Input: dimensioned drawing with shaded views. Units: mm. Origin: part minimum x, y, z. Coordinates: 2 decimals unless noted, no trailing zeros. Order: outer loops, then holes, each group sorted by start corner. A loop starts at its lowest first (then second) coordinate and runs counter-clockwise, first axis right, second up. Notation, with made-up numbers: (18, 77.25) -> (65, 77.25) arc R26 ccw to (65, 91.25) -> close; hole circle Ø10 at (56, 71.5). An arc over 180 degrees is marked (long way). Answer in a Markdown table with one row per item. Add a question column.
1) Section query C-C on z = 39. Return the cut outline in (x, y), then the cut area to 3 significant figures.
2) Pull-direction query (X, two-part tool) for the marked faces 1, 2, 3 and 4; classes: +X half, -X half, draft (parallel to the pull), parting line (faces both ways), or undercut.
3) Ray query, line 1 (X direction, y = 11.25, z = 5.5); line 2 (Y direction, x = 7, z = 32). Return the intervals inside material, ascending. Write a range as from..to.
4) Contact query for flat-ended pins moving along their axis: P1, Ø5, axis at x = 58.5, y = 10.5, coming from the +Z side; P2, Ø8, axis at x = 47.5, z = 70, coming from the +Y side; P3, Ø1.8, axis at x = 58, z = 21.5, coming from the +Y side. Output: stop coordinate, or through.
5) Section query D-D on y = 10.5. Return the cut outline in (x, z), then the cut area to 3 significant figures.
6) Section query A-A on y = 21. Return the cut outline in (x, z).
7) Section query B-B on x = 4.5. Return the cut outline in (y, z), then the cut area to 3 significant figures.
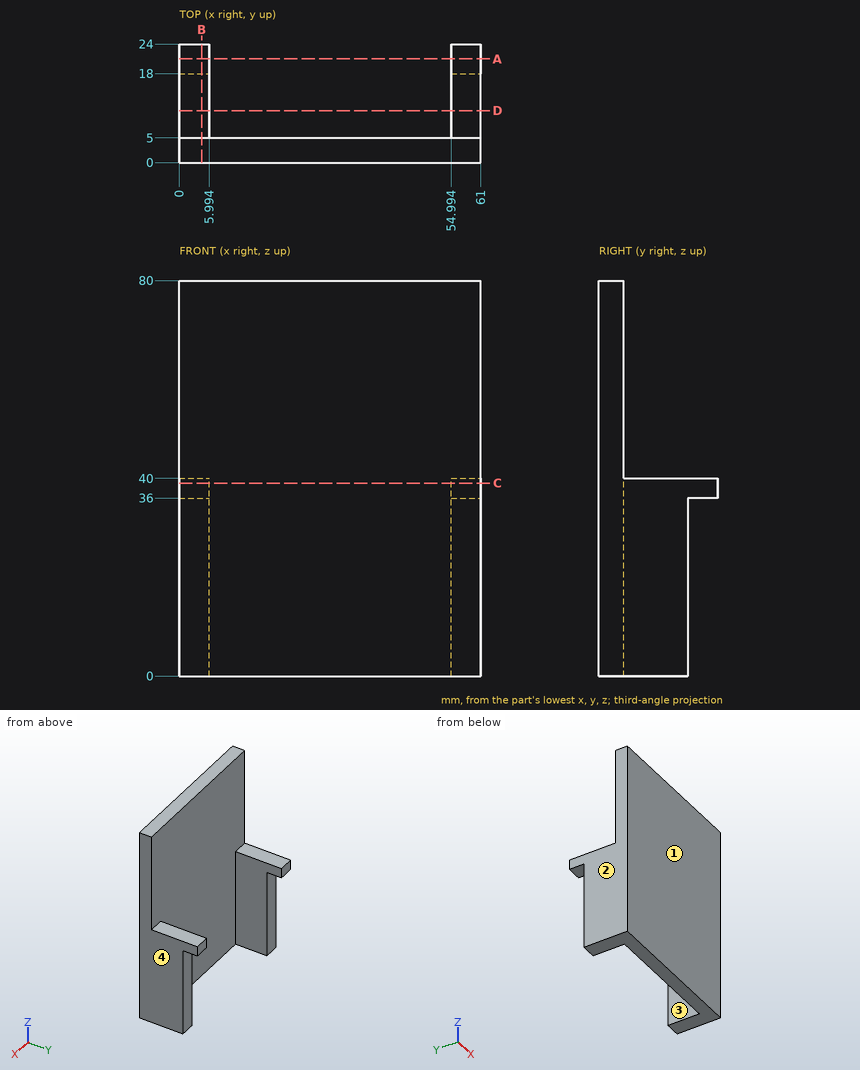
Result:
| question | item | result |
|---|---|---|
| 1 | outline | (0, 0) -> (61, 0) -> (61, 24) -> (54.99, 24) -> (54.99, 5) -> (5.99, 5) -> (5.99, 24) -> (0, 24) -> close |
| 1 | area | 533 mm2 |
| 2 | face 1 | draft |
| 2 | face 2 | -X half |
| 2 | face 3 | undercut |
| 2 | face 4 | +X half |
| 3 | line 1 | 0..5.99, 54.99..61 |
| 3 | line 2 | 0..5 |
| 4 | P1 | z = 40 |
| 4 | P2 | y = 5 |
| 4 | P3 | y = 18 |
| 5 | outline | (0, 0) -> (5.99, 0) -> (5.99, 40) -> (0, 40) -> close; (54.99, 0) -> (61, 0) -> (61, 40) -> (54.99, 40) -> close |
| 5 | area | 480 mm2 |
| 6 | outline | (0, 36) -> (5.99, 36) -> (5.99, 40) -> (0, 40) -> close; (54.99, 36) -> (61, 36) -> (61, 40) -> (54.99, 40) -> close |
| 7 | outline | (0, 0) -> (18, 0) -> (18, 36) -> (24, 36) -> (24, 40) -> (5, 40) -> (5, 80) -> (0, 80) -> close |
| 7 | area | 944 mm2 |
